Check sheet for the modelled part. Datum: model origin and axes. Units: mm. A direction names the side the tool comes from. Coordinates: 2 decimals unless noted, no trailing zeros. Loops run counter-clockwise (first coordinate to the right, second up) from the corner with the lowest first, then second, coordinate; pieces in that order, holes last. Notation, with made-up numbers: M -9.75,70.5 L 8.25,70.5 A14 cw 8.25,74.5 Z; hole C 88.5,-9 d1. An arc over 180 degrees is marked long. Use CSV: the item, a comma, the result in double quotes. Start each with the question number.
(1) Draft check along Z on faces 1 (the cylindrical face through (-1, 5, 0)), 2 (the flat face through (-1, 0, -2)), 3 (the cylindrical face through (-1.05, 4.28, 0.07)). Enter one of: pulls with the +Z half, pulls with the -Z half, needs draft (parallel to the pull), parting line crosses it, or undercut.
(2) Set-up check for faces 4 (the flat face through (-1, 0, 2)), 5 (the flat face through (-1, 1, 0)), 6 (the flat face through (-75, 0, 0)): record each of +Z, -Z, +X, -X, +Y, -Y from which the full face is reachable in a straight line by a thin tool's end or side.
(3) Scan lines: line 1 (Y direction, x = -25, z = -1.5); line 2 (Z direction, x = 60.5, y = -3.25); line 3 (Y direction, x = 19, z = 1). Record each from-to range of solid material in increasing order.
(4) Section check A-A on x = 53. Record the cut outline in (y, z).
(5) Go/stop test with flat-tipped pins: pin 1 Ø2 at (x, y) = (-9, -2.5) entering from +Z; pin 2 Ø1.8 at (x, z) = (-22, 2) entering from -Y; pin 3 Ø4 at (x, z) = (-31, -2.5) entering from -Y. Record where each tip stops, or that it passes through.
(6) Section check B-B on y = 3. Record the cut outline in (x, z).
from build123d import *

# Parameters (mm, degrees)
EXTRUDE_2_DEPTH      = 75
EXTRUDE_2_DEPTH_BACK = 75


with BuildPart() as part:
    # 草图1<2> → 凸台-拉伸2 (new, two sides: drawn at the far end of the back side and taken through both)
    with BuildSketch(Plane(origin=(0, 0, 0), x_dir=(0, 0, -1), z_dir=(1, 0, 0)).offset(-EXTRUDE_2_DEPTH_BACK)):
        with BuildLine():
            Line((-4, 0), (-0.5, 0))
            Line((-0.5, 0), (-0.5, -1.406748669))
            Line((-0.5, -1.406748669), (-1.219669914, -0.687078754))
            Line((-1.219669914, -0.687078754), (-1.75, -1.21740884))
            Line((-1.75, -1.21740884), (-0.5, -2.46740884))
            Line((-0.5, -2.46740884), (-0.5, -3.49335212))
            Line((-0.5, -3.49335212), (-1.219669914, -2.773682206))
            Line((-1.219669914, -2.773682206), (-1.75, -3.304012292))
            Line((-1.75, -3.304012292), (0, -5.054012292))
            Line((0, -5.054012292), (1.75, -3.304012292))
            Line((1.75, -3.304012292), (1.219669914, -2.773682206))
            Line((1.219669914, -2.773682206), (0.5, -3.49335212))
            Line((0.5, -3.49335212), (0.5, -2.46740884))
            Line((0.5, -2.46740884), (1.75, -1.21740884))
            Line((1.75, -1.21740884), (1.219669914, -0.687078754))
            Line((1.219669914, -0.687078754), (0.5, -1.406748669))
            Line((0.5, -1.406748669), (0.5, 0))
            Line((0.5, 0), (4, 0))
            Line((4, 0), (4, 1))
            ThreePointArc((4, 1), (0, 5), (-4, 1))
            Line((-4, 1), (-4, 0))
        make_face()
        with BuildLine():
            Line((3.282029094, 1), (-3.282029094, 1))
            ThreePointArc((-3.282029094, 1), (0, 4.282029094), (3.282029094, 1))
        make_face(mode=Mode.SUBTRACT)
    extrude(amount=EXTRUDE_2_DEPTH + EXTRUDE_2_DEPTH_BACK)


solid = part.part
Outcome:
1,face 1,"parting line crosses it"
1,face 2,"needs draft"
1,face 3,"undercut"
2,face 4,"+Z, +X, -X"
2,face 5,"+X, -X"
2,face 6,"+Z, -Z, -X, +Y, -Y"
3,line 1,"y = -3.55 to -3.05, -1.47 to -0.97, 0 to 1, 3.92 to 4.71"
3,line 2,"z = -1.7 to -0.74, -0.5 to 0.5, 0.74 to 1.7"
3,line 3,"y = -4.05 to -2.99, -1.97 to -0.91, 0 to 1, 4.13 to 4.87"
4,outline,"M -5.05,0 L -3.3,-1.75 L -2.77,-1.22 L -3.49,-0.5 L -2.47,-0.5 L -1.22,-1.75 L -0.69,-1.22 L -1.41,-0.5 L 0,-0.5 L 0,-4 L 1,-4 A4 ccw 1,4 L 0,4 L 0,0.5 L -1.41,0.5 L -0.69,1.22 L -1.22,1.75 L -2.47,0.5 L -3.49,0.5 L -2.77,1.22 L -3.3,1.75 Z; hole M 1,-3.28 A3.28 ccw 1,3.28 Z"
5,pin 1,"stops at z = 1.75"
5,pin 2,"stops at y = -3.95"
5,pin 3,"stops at y = -4.55"
6,outline,"M -75,-3.46 L 75,-3.46 L 75,-2.6 L -75,-2.6 Z; M -75,2.6 L 75,2.6 L 75,3.46 L -75,3.46 Z"
